Build history of the part. All positions in model axes, mm. Give positions to 0.01 mm unless a question says otherwise; leave off trailing zeros. Order: outer loops, then holes, each group sorted by start corner. A loop starts at its lowest first (then second) coordinate and runs counter-clockwise, first axis right, second up. Notation, with made-up numbers: (55, -18.5) -> (80, -18.5) arc R15 ccw to (80, 6.5) -> close; hole circle Ø8 at (52.5, -11.75). An arc over 180 degrees is marked (long way). Write item = value, one per line. Start each with the question number.
from build123d import *

# Parameters (mm, degrees)
SKETCH17_R                       = 3.4
ALUMINIUM_EXTRUSION_3030_1_DEPTH = 400


with BuildPart() as part:
    # Sketch17 → Aluminium extrusion 3030(1) (new body)
    with BuildSketch(Plane(origin=(0, 0, 0), x_dir=(0, 0, -1), z_dir=(1, 0, 0))):
        with BuildLine():
            Line((0, 6), (-4.302943725, 6))
            Line((-4.302943725, 6), (-8.3, 9.997056275))
            Line((-8.3, 9.997056275), (-8.3, 12.8))
            Line((-8.3, 12.8), (-4, 12.8))
            Line((-4, 12.8), (-4, 15))
            Line((-4, 15), (-13, 15))
            ThreePointArc((-13, 15), (-14.414213562, 14.414213562), (-15, 13))
            Line((-15, 13), (-15, 4))
            Line((-15, 4), (-12.8, 4))
            Line((-12.8, 4), (-12.8, 8.3))
            Line((-12.8, 8.3), (-9.997056275, 8.3))
            Line((-9.997056275, 8.3), (-6, 4.302943725))
            Line((-6, 4.302943725), (-6, 0))
            Line((-6, 0), (-6, -4.302943725))
            Line((-6, -4.302943725), (-9.997056275, -8.3))
            Line((-9.997056275, -8.3), (-12.8, -8.3))
            Line((-12.8, -8.3), (-12.8, -4))
            Line((-12.8, -4), (-15, -4))
            Line((-15, -4), (-15, -13))
            ThreePointArc((-15, -13), (-14.414213562, -14.414213562), (-13, -15))
            Line((-13, -15), (-4, -15))
            Line((-4, -15), (-4, -12.8))
            Line((-4, -12.8), (-8.3, -12.8))
            Line((-8.3, -12.8), (-8.3, -9.997056275))
            Line((-8.3, -9.997056275), (-4.302943725, -6))
            Line((-4.302943725, -6), (0, -6))
            Line((0, -6), (4.302943725, -6))
            Line((4.302943725, -6), (8.3, -9.997056275))
            Line((8.3, -9.997056275), (8.3, -12.8))
            Line((8.3, -12.8), (4, -12.8))
            Line((4, -12.8), (4, -15))
            Line((4, -15), (13, -15))
            ThreePointArc((13, -15), (14.414213562, -14.414213562), (15, -13))
            Line((15, -13), (15, -4))
            Line((15, -4), (12.8, -4))
            Line((12.8, -4), (12.8, -8.3))
            Line((12.8, -8.3), (9.997056275, -8.3))
            Line((9.997056275, -8.3), (6, -4.302943725))
            Line((6, -4.302943725), (6, 0))
            Line((6, 0), (6, 4.302943725))
            Line((6, 4.302943725), (9.997056275, 8.3))
            Line((9.997056275, 8.3), (12.8, 8.3))
            Line((12.8, 8.3), (12.8, 4))
            Line((12.8, 4), (15, 4))
            Line((15, 4), (15, 13))
            ThreePointArc((15, 13), (14.414213562, 14.414213562), (13, 15))
            Line((13, 15), (4, 15))
            Line((4, 15), (4, 12.8))
            Line((4, 12.8), (8.3, 12.8))
            Line((8.3, 12.8), (8.3, 9.997056275))
            Line((8.3, 9.997056275), (4.302943725, 6))
            Line((4.302943725, 6), (0, 6))
        make_face()
        Circle(SKETCH17_R, mode=Mode.SUBTRACT)
    extrude(amount=ALUMINIUM_EXTRUSION_3030_1_DEPTH)


solid = part.part
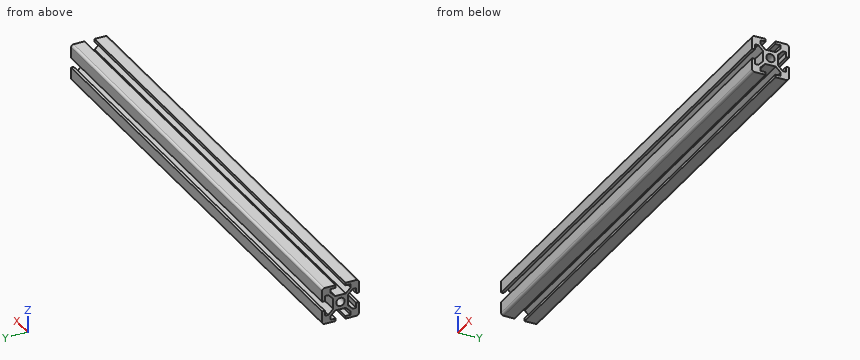
(1) Flat gauge pin, fed straight in: P1, Ø4.5, axis at x = 111.5, y = 1.5, coming from the -Z side. Where does the tip first touch, or does it go through?
(2) Cut at A-A, the plane z = 0. Give the cut face in (x, y), plus the area to 3 significant figures.
(3) Wall check: line 1 (Z direction, x = 173.5, y = -12); line 2 (Y direction, x = 145, z = 0). Give the ranges that are in metal, low to high. Write a range as [from, to].
Results:
q1.P1 = -6
q2.outline = (0, -6) -> (400, -6) -> (400, -3.4) -> (0, -3.4) -> close; (0, 3.4) -> (400, 3.4) -> (400, 6) -> (0, 6) -> close
q2.area = 2,080 mm2
q3.line_1 = [-15, -8.3], [8.3, 15]
q3.line_2 = [-6, -3.4], [3.4, 6]
